The drawing under review shows one solid part. Ordinate dimensions are in mm from its lowest x, y, z. A direction names the side the tool comes from. Round coordinates to 2 decimals unless told otherwise and drop trailing zeros. Order: outer loops, then holes, each group sorted by start corner. A loop starts at its lowest first (then second) coordinate and runs counter-clockwise, first axis right, second up. Notation, with made-up numbers: M 47,75 L 99,75 A22 cw 99,109 Z; hole C 83.5,3 d11. An arc over 180 degrees is marked long. Answer as a JSON object with one key per item and string values. Group by question number.
1) Consider section C-C, the plane x = 127. Write out the cut boundary in (y, z).
2) Consider section D-D, the plane x = 168.5. Write out the cut boundary in (y, z), then the cut area to 3 significant figures.
3) The part is to be moulded in two halves that separate along Y. For the marked faces 1, 2, 3 and 4, say which applies: +Y half, -Y half, draft (parallel to the pull), parting line (faces both ways), or undercut.
4) To check wall thickness, follow line 1 (X direction, y = 50, z = 8); line 2 (Y direction, x = 127, z = 6); line 3 (Z direction, x = 75, y = 119). State the ranges of each line that lie inside material, in increasing order.
5) Insertion check: pin 1 Ø4 at (y, z) = (74.5, 11) entering from -X; pin 2 Ø12.5 at (x, z) = (37.5, 36) entering from +Y; pin 3 Ø3 at (y, z) = (65, 28.5) entering from +X; pin 4 Ø7.5 at (y, z) = (96, 34) entering from -X. Each pin has a flat end and moves straight along its axis. Give the tip position at first contact, or say it passes through.
6) Consider section A-A, the plane y = 43.5. Write out the cut boundary in (x, z), then the cut area to 3 significant figures.
7) For the marked faces 5 and 6, list the 3-axis set-ups (+Z, -Z, +X, -X, +Y, -Y) from which the entire face can be reached by the end or side of a thin tool; tool diameter is ignored.
8) Consider section B-B, the plane z = 30.5. Write out the cut boundary in (x, y), then the cut area to 3 significant figures.
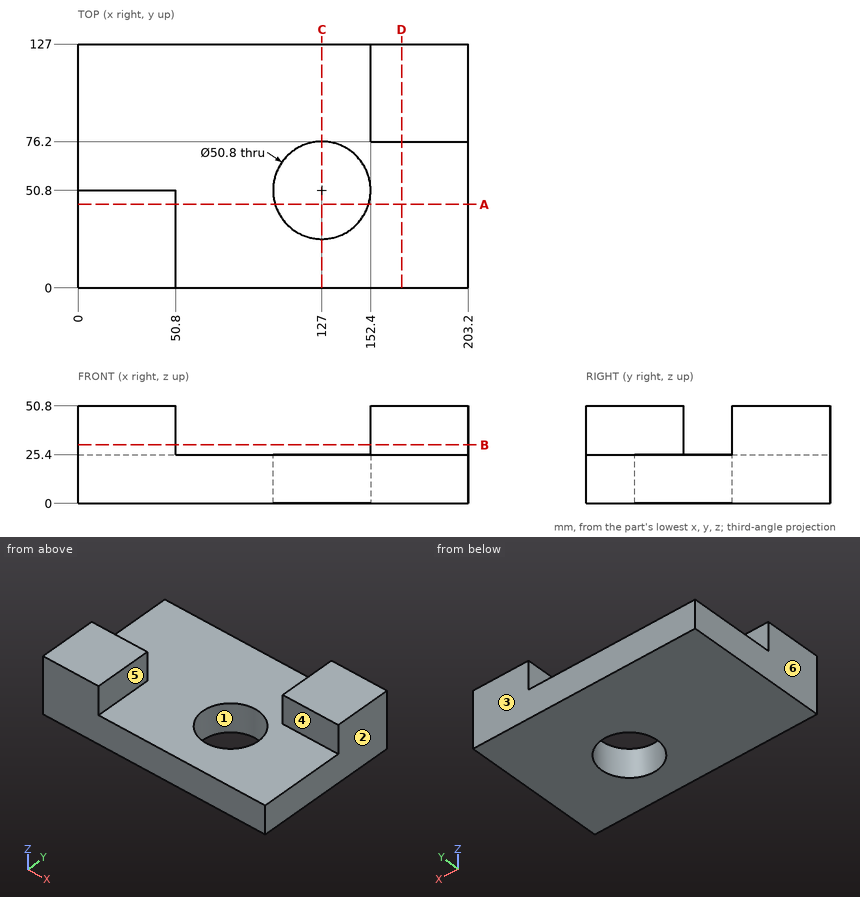
Results list:
{
 "1": {"outline": "M 0,0 L 25.4,0 L 25.4,25.4 L 0,25.4 Z; M 76.2,0 L 127,0 L 127,25.4 L 76.2,25.4 Z"},
 "2": {"outline": "M 0,0 L 127,0 L 127,50.8 L 76.2,50.8 L 76.2,25.4 L 0,25.4 Z", "area": "4,520 mm^2"},
 "3": {"face 1": "undercut", "face 2": "draft", "face 3": "+Y half", "face 4": "-Y half"},
 "4": {"line 1": "0 to 101.61, 152.39 to 203.2", "line 2": "0 to 25.4, 76.2 to 127", "line 3": "0 to 25.4"},
 "5": {"pin 1": "x = 0", "pin 2": "y = 50.8", "pin 3": "through", "pin 4": "x = 152.4"},
 "6": {"outline": "M 0,0 L 102.67,0 L 102.67,25.4 L 50.8,25.4 L 50.8,50.8 L 0,50.8 Z; M 151.33,0 L 203.2,0 L 203.2,25.4 L 151.33,25.4 Z", "area": "5,220 mm^2"},
 "7": {"face 5": "+Z, +X, +Y, -Y", "face 6": "+Z, -Z, -X, +Y, -Y"},
 "8": {"outline": "M 0,0 L 50.8,0 L 50.8,50.8 L 0,50.8 Z; M 152.4,76.2 L 203.2,76.2 L 203.2,127 L 152.4,127 Z", "area": "5,160 mm^2"}
}
